For this review, take the finished solid that the model builds, in its own axes (mm). Round coordinates to 2 decimals unless told otherwise and drop trailing zeros. Write each loop counter-clockwise with the first axis right and the second up, starting at its lowest first coordinate (ties: lowest second). Pieces come first, ordered by that corner, then holes. Notation, with made-up numbers: (58, 61) -> (93, 61) arc R17 ccw to (93, 94) -> close; hole circle Ø1 at (10.5, 46.25). An arc over 180 degrees is marked (long way). Write item = value, one per line. Start each with the question number.
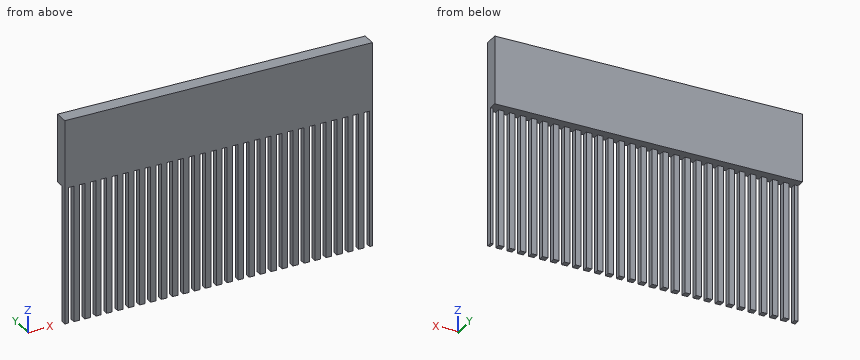
```python
from build123d import *

# Parameters (mm, degrees)
SKETCH1_W           = 115
SKETCH1_H           = 15
BOSS_EXTRUDE1_DEPTH = 0.5
SKETCH2_W           = 115
SKETCH2_H           = 10
CUT_EXTRUDE1_DEPTH  = 0.1
SKETCH3_W           = 0.4
SKETCH3_H           = 10
CUT_EXTRUDE2_DEPTH  = 0.4
LPATTERN3_COUNT     = 150
LPATTERN3_PITCH     = 0.8
SKETCH4_W           = 115
SKETCH4_H           = 5
BOSS_EXTRUDE2_DEPTH = 1
SKETCH5_W           = 77.289086501
SKETCH5_H           = 15.822063322
CUT_EXTRUDE3_DEPTH  = 1
SKETCH6_W           = 3.197112069
SKETCH6_H           = 15.066627115
CUT_EXTRUDE4_DEPTH  = 1
SKETCH7_W           = 12.052245582
SKETCH7_H           = 15.126214191
CUT_EXTRUDE5_DEPTH  = 10


with BuildPart() as part:
    # Sketch1 → Boss-Extrude1 (new body)
    with BuildSketch(Plane(origin=(0, 0, 0), x_dir=(1, 0, 0), z_dir=(0, 1, 0))):
        with Locations((57.5, 7.5)):
            Rectangle(SKETCH1_W, SKETCH1_H)
    extrude(amount=BOSS_EXTRUDE1_DEPTH)

    # Sketch2 → Cut-Extrude1 (cut)
    with BuildSketch(Plane(origin=(0, 0.5, 0), x_dir=(1, 0, 0), z_dir=(0, 1, 0))):
        with Locations((57.5, 10)):
            Rectangle(SKETCH2_W, SKETCH2_H)
    extrude(amount=-CUT_EXTRUDE1_DEPTH, mode=Mode.SUBTRACT)

    # Sketch3 → Cut-Extrude2 (cut)
    with BuildSketch(Plane(origin=(0, 0.4, 0), x_dir=(1, 0, 0), z_dir=(0, 1, 0))):
        with Locations((0.2, 10)):
            Rectangle(SKETCH3_W, SKETCH3_H)
    cut_extrude2 = extrude(amount=-CUT_EXTRUDE2_DEPTH, mode=Mode.SUBTRACT)

    # LPattern3: Cut-Extrude2 ×150
    with Locations(*[(i * LPATTERN3_PITCH, 0, 0) for i in range(1, LPATTERN3_COUNT)]):
        add(cut_extrude2, mode=Mode.SUBTRACT)

    # Sketch4 → Boss-Extrude2 (add)
    with BuildSketch(Plane.XZ):
        with Locations((57.5, -2.5)):
            Rectangle(SKETCH4_W, SKETCH4_H)
    extrude(amount=-BOSS_EXTRUDE2_DEPTH)

    # Sketch5 → Cut-Extrude3 (cut)
    with BuildSketch(Plane(origin=(0, 1, 0), x_dir=(1, 0, 0), z_dir=(0, 1, 0))):
        with Locations((38.64454325, 7.911031661)):
            Rectangle(SKETCH5_W, SKETCH5_H)
    extrude(amount=-CUT_EXTRUDE3_DEPTH, mode=Mode.SUBTRACT)

    # Sketch6 → Cut-Extrude4 (cut)
    with BuildSketch(Plane(origin=(0, 1, 0), x_dir=(1, 0, 0), z_dir=(0, 1, 0))):
        with Locations((78.887642535, 7.533313558)):
            Rectangle(SKETCH6_W, SKETCH6_H)
    extrude(amount=-CUT_EXTRUDE4_DEPTH, mode=Mode.SUBTRACT)

    # Sketch7 → Cut-Extrude5 (cut)
    with BuildSketch(Plane(origin=(0, 1, 0), x_dir=(1, 0, 0), z_dir=(0, 1, 0))):
        with Locations((86.512321361, 7.563107096)):
            Rectangle(SKETCH7_W, SKETCH7_H)
    extrude(amount=-CUT_EXTRUDE5_DEPTH, mode=Mode.SUBTRACT)


solid = part.part
```
1. Wall thickness on L1, parallel to Y at x = 109.5, z = -12.5; L2, parallel to Z at x = 103, y = 0.85: over which ranges is each line inside the solid? List them lowest first. Write a range as from..to.
2. Consider section A-A, the plane z = -7.5. Give the number of separate pieces and of enclosed holes in the cut face, then the cut area to 3 significant figures.
3. Clearance check with a flat-ended pin moving along its axis: pin 1 Ø2 at (x, z) = (97, -13) entering from -Y. State where the tip first meets the part, or that it passes through.
4. Consider section B-B, the plane y = 0.8. Give the boundary of the cut face in (x, z).
Outcome:
q1.L1 = 0..0.4
q1.L2 = -5..0
q2.separate_pieces = 29
q2.enclosed_holes = 0
q2.area = 4.50 mm2
q3.pin_1 = 0
q4.outline = (92.54, -5) -> (115, -5) -> (115, 0) -> (92.54, 0) -> close
